For this review, use the dimensioned drawing (mm, ordinates from the lowest corner) and the shaded views. A direction names the side the tool comes from. Coordinates: 2 decimals unless noted, no trailing zeros. Write each loop counter-clockwise with the first axis right and the second up, starting at its lowest first coordinate (ties: lowest second). Pieces come first, ordered by that corner, then holes.
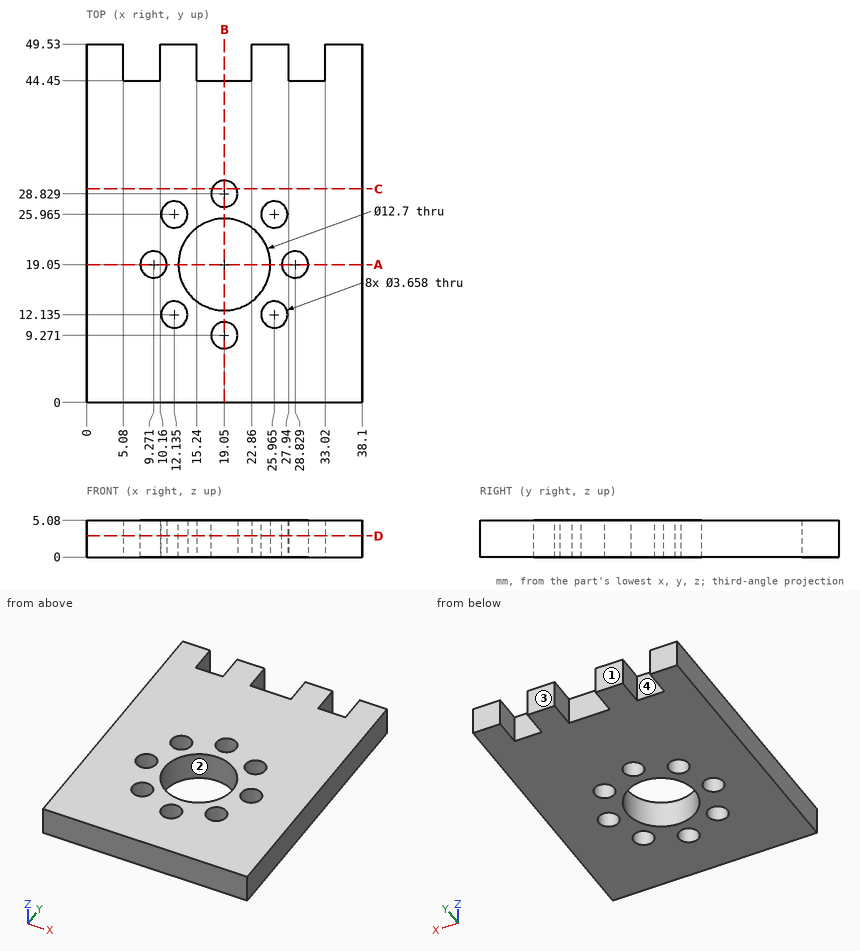
Item 1: Mouldability with a two-part tool opening along X and no side actions: class the marked faces 1 and 2 as pulls with the +X half, pulls with the -X half, needs draft (parallel to the pull), parting line crosses it, or undercut.
Solved:
face 1: needs draft
face 2: undercut
Item 2: For pin 1 (2 mm diameter, centred on x = 28.829, y = 19.05, fed in from +Z); pin 2 (2.5 mm diameter, centred on x = 31, z = 3, fed in from +Y), all flat-tipped, find the tip position at first contact; note any pin that passes through.
Solved:
pin 1: passes through
pin 2: stops at y = 44.45
Item 3: To check wall thickness, follow line 1 along Y through (x, z) = (12, 4.45); line 2 along Y through (x, z) = (19.05, 3.2); line 3 along X through (y, z) = (47, 2.65). State the ranges of each line that lie inside material, in increasing order.
Solved:
line 1: y = 0 to 10.31, 13.96 to 24.14, 27.79 to 49.53
line 2: y = 0 to 7.44, 11.1 to 12.7, 25.4 to 27, 30.66 to 44.45
line 3: x = 0 to 5.08, 10.16 to 15.24, 22.86 to 27.94, 33.02 to 38.1
Item 4: Take a section at C-C, the plane y = 29.5. Write out the cut boundary in (x, z).
Solved:
outline: (0, 0) - (17.35, 0) - (17.35, 5.08) - (0, 5.08) - close; (20.75, 0) - (38.1, 0) - (38.1, 5.08) - (20.75, 5.08) - close
Item 5: Take a section at D-D, the plane z = 2.95. Count the separate pieces of the cut face and the enclosed holes in it, plus the area to 3 significant figures.
Solved:
separate pieces: 1
enclosed holes: 9
area: 1,590 mm2
Item 6: Machinability: for the marked faces 3 and 4, which of the approach directions +Z, -Z, +X, -X, +Y, -Y give a long, thin tool a straight path to every point of the face, cutting with its end or side? Answer none if there is none.
Solved:
face 3: +Z, -Z, +X, -X, +Y
face 4: +Z, -Z, +Y
Item 7: Take a section at B-B, the plane x = 19.05. Write out the cut boundary in (y, z), plus the area to 3 significant figures.
Solved:
outline: (0, 0) - (7.44, 0) - (7.44, 5.08) - (0, 5.08) - close; (11.1, 0) - (12.7, 0) - (12.7, 5.08) - (11.1, 5.08) - close; (25.4, 0) - (27, 0) - (27, 5.08) - (25.4, 5.08) - close; (30.66, 0) - (44.45, 0) - (44.45, 5.08) - (30.66, 5.08) - close
area: 124 mm2
Item 8: Take a section at A-A, the plane y = 19.05. Write out the cut boundary in (x, z).
Solved:
outline: (0, 0) - (7.44, 0) - (7.44, 5.08) - (0, 5.08) - close; (11.1, 0) - (12.7, 0) - (12.7, 5.08) - (11.1, 5.08) - close; (25.4, 0) - (27, 0) - (27, 5.08) - (25.4, 5.08) - close; (30.66, 0) - (38.1, 0) - (38.1, 5.08) - (30.66, 5.08) - close
